The model under review builds one solid part; all positions refer to its coordinate system, in mm. A direction names the side the tool comes from. Round coordinates to 2 decimals unless told otherwise and drop trailing zeros. Write each loop counter-clockwise with the first axis right and the second up, starting at its lowest first coordinate (ties: lowest second). Pieces come first, ordered by that corner, then holes. Notation, with made-up numbers: (-21, -16.75) -> (28, -16.75) arc R31 ccw to (28, 16.25) -> close; hole circle Ø8 at (7, 68). An arc over 180 degrees is marked (long way). Return JSON: item names as keys, results as strings. Group by question number.
1. Tool access review of faces 1 (the flat face through (52.986, -0.07, 6.789)), 2 (the flat face through (-6.528, -0.14, 15.578)), 3 (the flat face through (26.57, -0.06, 5.65)): name each direction out of +Z, -Z, +X, -X, +Y, -Y from which nothing blocks a thin tool from reaching the whole face with its end or side.
2. Clearance check with flat-ended pins moving along their axes: P1, Ø1.6, axis at x = 10.5, y = 1.5, coming from the +Z side; P2, Ø1.9, axis at x = 64.5, z = 4.5, coming from the -Y side; P3, Ø5, axis at x = 26, z = 9.5, coming from the +Y side. State where each tip first meets the part, or that it passes through.
3. Take a section at A-A, the plane z = 11.75. Give the number of separate pieces and of enclosed holes in the cut face, then the cut area to 3 significant figures.
4. Take a section at B-B, the plane z = 19.75. Write out the cut boundary in (x, y), then the cut area to 3 significant figures.
5. For line 1 along X through (y, z) = (-8.5, 4.5); line 2 along Y through (x, z) = (-8.95, 7); line 3 along X through (y, z) = (0.25, 20), list the stretches that pass through material, from the lowest coordinate up. Write a range as from..to.
6. Mouldability with a two-part tool opening along Y and no side actions: class faces 4 (the flat face through (20, -5, 4)), 5 (the flat face through (10, 0, 6)), 6 (the flat face through (76.949, -0.126, 14.215)), 7 (the flat face through (80, 9, 8)) as pulls with the +Y half, pulls with the -Y half, needs draft (parallel to the pull), parting line crosses it, or undercut.
from build123d import *

# Parameters (mm, degrees)
SKETCH1_W            = 20
SKETCH1_H            = 20
BOSS_EXTRUDE1_DEPTH  = 10
SKETCH2_W            = 4
SKETCH2_H            = 10
BOSS_EXTRUDE2_DEPTH  = 20
SKETCH3_W            = 10
SKETCH3_H            = 20
BOSS_EXTRUDE3_DEPTH  = 20
SKETCH4_W            = 4
SKETCH4_H            = 10
BOSS_EXTRUDE4_DEPTH  = 20
SKETCH5_W            = 10
SKETCH5_H            = 20
BOSS_EXTRUDE5_DEPTH  = 20
BOSS_EXTRUDE6_DEPTH  = 20
BOSS_EXTRUDE7_DEPTH  = 20
BOSS_EXTRUDE8_DEPTH  = 10
SKETCH9_R            = 1.45
CUT_EXTRUDE1_DEPTH   = 1.5
SKETCH10_W           = 8
SKETCH10_H           = 18
CUT_EXTRUDE2_DEPTH   = 17
SKETCH13_W           = 8
SKETCH13_H           = 18
CUT_EXTRUDE4_DEPTH   = 19
SKETCH14_W           = 10
SKETCH14_H           = 20
BOSS_EXTRUDE9_DEPTH  = 1
SKETCH15_W           = 8
SKETCH15_H           = 18
CUT_EXTRUDE5_DEPTH   = 19
SKETCH16_W           = 10
SKETCH16_H           = 20
BOSS_EXTRUDE10_DEPTH = 1
SKETCH12_W           = 2
SKETCH12_H           = 8
CUT_EXTRUDE3_DEPTH   = 80
CUT_EXTRUDE7_DEPTH   = 19
SKETCH19_W           = 5.878679656
SKETCH19_H           = 18
CUT_EXTRUDE8_DEPTH   = 5
BOSS_EXTRUDE12_DEPTH = 1
CUT_EXTRUDE10_DEPTH  = 9
SKETCH23_W           = 2.302943726
SKETCH23_H           = 8
CUT_EXTRUDE11_DEPTH  = 3
BOSS_EXTRUDE13_DEPTH = 1
FILLET3_R            = 2
FILLET4_R            = 2


with BuildPart() as part:
    # Sketch1 → Boss-Extrude1 (new body)
    with BuildSketch(Plane.XY):
        Rectangle(SKETCH1_W, SKETCH1_H)
    extrude(amount=BOSS_EXTRUDE1_DEPTH)

    # Sketch2 → Boss-Extrude2 (add)
    with BuildSketch(Plane(origin=(10, 0, 0), x_dir=(0, 0, -1), z_dir=(1, 0, 0))):
        with Locations((-2, 0)):
            Rectangle(SKETCH2_W, SKETCH2_H)
    extrude(amount=BOSS_EXTRUDE2_DEPTH)

    # Sketch3 → Boss-Extrude3 (add)
    with BuildSketch(Plane(origin=(30, 0, 0), x_dir=(0, 0, -1), z_dir=(1, 0, 0))):
        with Locations((-5, 0)):
            Rectangle(SKETCH3_W, SKETCH3_H)
    extrude(amount=BOSS_EXTRUDE3_DEPTH)

    # Sketch4 → Boss-Extrude4 (add)
    with BuildSketch(Plane(origin=(50, 0, 0), x_dir=(0, 0, -1), z_dir=(1, 0, 0))):
        with Locations((-2, 0)):
            Rectangle(SKETCH4_W, SKETCH4_H)
    extrude(amount=BOSS_EXTRUDE4_DEPTH)

    # Sketch5 → Boss-Extrude5 (add)
    with BuildSketch(Plane(origin=(70, 0, 0), x_dir=(0, 0, -1), z_dir=(1, 0, 0))):
        with Locations((-5, 0)):
            Rectangle(SKETCH5_W, SKETCH5_H)
    extrude(amount=BOSS_EXTRUDE5_DEPTH)

    # Sketch6 → Boss-Extrude6 (add)
    with BuildSketch(Plane.XZ.offset(10)):
        Polygon((-8.5, 10), (-4.5, 21.313708499), (-0.5, 10), align=None)
        Polygon((9, 10), (1, 10), (5, 21.313708499), align=None)
    extrude(amount=-BOSS_EXTRUDE6_DEPTH)

    # Sketch7 → Boss-Extrude7 (add)
    with BuildSketch(Plane.XZ.offset(10)):
        Polygon((31.5, 10), (35.5, 21.313708499), (39.5, 10), align=None)
        Polygon((71.5, 10), (75.5, 21.313708499), (79.5, 10), align=None)
        Polygon((41, 10), (49, 10), (45, 21.313708499), align=None)
        Polygon((81, 10), (89, 10), (85, 21.313708499), align=None)
    extrude(amount=-BOSS_EXTRUDE7_DEPTH)

    # Sketch8 → Boss-Extrude8 (add)
    with BuildSketch(Plane.XZ.offset(5)):
        Polygon((12, 4), (14, 9.656854249), (16, 4), align=None)
        Polygon((52, 4), (54, 9.656854249), (56, 4), align=None)
        Polygon((18, 4), (22, 4), (20, 9.656854249), align=None)
        Polygon((58, 4), (62, 4), (60, 9.656854249), align=None)
        Polygon((24, 4), (28, 4), (26, 9.656854249), align=None)
        Polygon((64, 4), (68, 4), (66, 9.656854249), align=None)
    extrude(amount=-BOSS_EXTRUDE8_DEPTH)

    # Sketch9 → Cut-Extrude1 (cut)
    with BuildSketch(Plane.ZY.offset(10)):
        with Locations((7, 0)):
            Circle(SKETCH9_R)
    extrude(amount=-CUT_EXTRUDE1_DEPTH, mode=Mode.SUBTRACT)

    # Sketch10 → Cut-Extrude2 (cut)
    with BuildSketch(Plane.ZY.offset(8.5)):
        with Locations((5, 0)):
            Rectangle(SKETCH10_W, SKETCH10_H)
    extrude(amount=-CUT_EXTRUDE2_DEPTH, mode=Mode.SUBTRACT)

    # Sketch13 → Cut-Extrude4 (cut)
    with BuildSketch(Plane.ZY.offset(-30)):
        with Locations((5, 0)):
            Rectangle(SKETCH13_W, SKETCH13_H)
    extrude(amount=-CUT_EXTRUDE4_DEPTH, mode=Mode.SUBTRACT)

    # Sketch14 → Boss-Extrude9 (add)
    with BuildSketch(Plane.ZY.offset(-30)):
        with Locations((5, 0)):
            Rectangle(SKETCH14_W, SKETCH14_H)
    extrude(amount=-BOSS_EXTRUDE9_DEPTH)

    # Sketch15 → Cut-Extrude5 (cut)
    with BuildSketch(Plane.ZY.offset(-70)):
        with Locations((5, 0)):
            Rectangle(SKETCH15_W, SKETCH15_H)
    extrude(amount=-CUT_EXTRUDE5_DEPTH, mode=Mode.SUBTRACT)

    # Sketch16 → Boss-Extrude10 (add)
    with BuildSketch(Plane.ZY.offset(-70)):
        with Locations((5, 0)):
            Rectangle(SKETCH16_W, SKETCH16_H)
    extrude(amount=-BOSS_EXTRUDE10_DEPTH)

    # Sketch12 → Cut-Extrude3 (cut)
    with BuildSketch(Plane.ZY.offset(-8.5)):
        with Locations((2, 0)):
            Rectangle(SKETCH12_W, SKETCH12_H)
    extrude(amount=-CUT_EXTRUDE3_DEPTH, mode=Mode.SUBTRACT)

    # Sketch17 → Cut-Extrude7 (cut)
    with BuildSketch(Plane.XZ.offset(10)):
        Polygon((-7.439339828, 10), (-4.5, 18.313708499), (-1.560660172, 10), align=None)
        Polygon((32.560660172, 10), (35.5, 18.313708499), (38.439339828, 10), align=None)
        Polygon((72.560660172, 10), (75.5, 18.313708499), (78.439339828, 10), align=None)
        Polygon((7.939339828, 10), (2.060660172, 10), (5, 18.313708499), align=None)
        Polygon((47.939339828, 10), (42.060660172, 10), (45, 18.313708499), align=None)
        Polygon((87.939339828, 10), (82.060660172, 10), (85, 18.313708499), align=None)
    extrude(amount=-CUT_EXTRUDE7_DEPTH, mode=Mode.SUBTRACT)

    # Sketch19 → Cut-Extrude8 (cut)
    with BuildSketch(Plane.XY.offset(10)):
        with Locations((-4.5, 0)):
            Rectangle(SKETCH19_W, SKETCH19_H)
        with Locations((35.5, 0)):
            Rectangle(SKETCH19_W, SKETCH19_H)
        with Locations((75.5, 0)):
            Rectangle(SKETCH19_W, SKETCH19_H)
        with Locations((5, 0)):
            Rectangle(SKETCH19_W, SKETCH19_H)
        with Locations((45, 0)):
            Rectangle(SKETCH19_W, SKETCH19_H)
        with Locations((85, 0)):
            Rectangle(SKETCH19_W, SKETCH19_H)
    extrude(amount=-CUT_EXTRUDE8_DEPTH, mode=Mode.SUBTRACT)

    # Sketch21 → Boss-Extrude12 (add)
    with BuildSketch(Plane.XZ.offset(10)):
        Polygon((-8.5, 10), (-4.5, 21.313708499), (-0.5, 10), align=None)
        Polygon((31.5, 10), (35.5, 21.313708499), (39.5, 10), align=None)
        Polygon((71.5, 10), (75.5, 21.313708499), (79.5, 10), align=None)
        Polygon((9, 10), (1, 10), (5, 21.313708499), align=None)
        Polygon((49, 10), (41, 10), (45, 21.313708499), align=None)
        Polygon((81, 10), (89, 10), (85, 21.313708499), align=None)
    extrude(amount=-BOSS_EXTRUDE12_DEPTH)

    # Sketch22 → Cut-Extrude10 (cut)
    with BuildSketch(Plane.XZ.offset(5)):
        Polygon((12.848528137, 4), (14, 7.256854249), (15.151471863, 4), align=None)
        Polygon((52.848528137, 4), (54, 7.256854249), (55.151471863, 4), align=None)
        Polygon((21.151471863, 4), (18.848528137, 4), (20, 7.256854249), align=None)
        Polygon((61.151471863, 4), (58.848528137, 4), (60, 7.256854249), align=None)
        Polygon((27.151471863, 4), (24.848528137, 4), (26, 7.256854249), align=None)
        Polygon((67.151471863, 4), (64.848528137, 4), (66, 7.256854249), align=None)
    extrude(amount=-CUT_EXTRUDE10_DEPTH, mode=Mode.SUBTRACT)

    # Sketch23 → Cut-Extrude11 (cut)
    with BuildSketch(Plane.XY.offset(4)):
        with Locations((14, 0)):
            Rectangle(SKETCH23_W, SKETCH23_H)
        with Locations((54, 0)):
            Rectangle(SKETCH23_W, SKETCH23_H)
        with Locations((20, 0)):
            Rectangle(SKETCH23_W, SKETCH23_H)
        with Locations((60, 0)):
            Rectangle(SKETCH23_W, SKETCH23_H)
        with Locations((26, 0)):
            Rectangle(SKETCH23_W, SKETCH23_H)
        with Locations((66, 0)):
            Rectangle(SKETCH23_W, SKETCH23_H)
    extrude(amount=-CUT_EXTRUDE11_DEPTH, mode=Mode.SUBTRACT)

    # Sketch24 → Boss-Extrude13 (add)
    with BuildSketch(Plane.XZ.offset(5)):
        Polygon((12, 4), (14, 9.656854249), (16, 4), align=None)
        Polygon((52, 4), (54, 9.656854249), (56, 4), align=None)
        Polygon((22, 4), (18, 4), (20, 9.656854249), align=None)
        Polygon((62, 4), (58, 4), (60, 9.656854249), align=None)
        Polygon((28, 4), (24, 4), (26, 9.656854249), align=None)
        Polygon((68, 4), (64, 4), (66, 9.656854249), align=None)
    extrude(amount=-BOSS_EXTRUDE13_DEPTH)

    # Fillet3
    fillet3_edges = [part.edges().sort_by_distance(p)[0] for p in [
        (10, -5, 2),
    ]]
    fillet(fillet3_edges, radius=FILLET3_R)

    # Fillet4
    fillet4_edges = [part.edges().sort_by_distance(p)[0] for p in [
        (30, 5, 2),
        (50, 5, 2),
        (10, 5, 2),
        (70, 5, 2),
        (50, -5, 2),
        (70, -5, 2),
        (30, -5, 2),
    ]]
    fillet(fillet4_edges, radius=FILLET4_R)


solid = part.part
Output:
{
 "1": {"face 1": "+Z, +Y, -Y", "face 2": "+Z, -X, +Y, -Y", "face 3": "none"},
 "2": {"P1": "stops at z = 10", "P2": "stops at y = -5", "P3": "stops at y = 5"},
 "3": {"separate pieces": "6", "enclosed holes": "6", "area": "310 mm^2"},
 "4": {"outline": "(-5.05, -10) -> (-3.95, -10) -> (-3.95, 10) -> (-5.05, 10) -> close; (4.45, -10) -> (5.55, -10) -> (5.55, 10) -> (4.45, 10) -> close; (34.95, -10) -> (36.05, -10) -> (36.05, 10) -> (34.95, 10) -> close; (44.45, -10) -> (45.55, -10) -> (45.55, 10) -> (44.45, 10) -> close; (74.95, -10) -> (76.05, -10) -> (76.05, 10) -> (74.95, 10) -> close; (84.45, -10) -> (85.55, -10) -> (85.55, 10) -> (84.45, 10) -> close", "area": "133 mm^2"},
 "5": {"line 1": "x = -10..-8.5, 8.5..10, 30..31, 49..50, 70..71, 89..90", "line 2": "y = -10..-1.45, 1.45..10", "line 3": "x = -4.96..-4.04, 4.54..5.46, 35.04..35.96, 44.54..45.46, 75.04..75.96, 84.54..85.46"},
 "6": {"face 4": "pulls with the -Y half", "face 5": "needs draft", "face 6": "undercut", "face 7": "undercut"}
}
